Geometry: final body of the model. Coordinates: model frame, mm. Face numbers are marked on the shaded views. A direction names the side the tool comes from. Round coordinates to 2 decimals unless told otherwise and drop trailing zeros. Loops run counter-clockwise (first coordinate to the right, second up) from the corner with the lowest first, then second, coordinate; pieces in that order, holes last. Notation, with made-up numbers: M -8,85.25 L 22,85.25 A15 ccw 22,95.25 Z; hole C -32.75,77.5 d7. An arc over 180 degrees is marked long. Answer as a JSON object with one key per item and string values.
from build123d import *

# Parameters (mm, degrees)
BASPROSKE_W         = 4
BASPROSKE_H         = 22.5
TOOTHCUT_DEPTH      = 33.070235422
TEETHCUTS_COUNT     = 18
TEETHCUTS_ANGLE     = 340
BORSKE_R            = 1.5
BORE_DEPTH          = 50.0000508
SKETCH_1_R          = 1.5
CUT_EXTRUDE_1_DEPTH = 32.895398001


with BuildPart() as part:
    # BasProSke → Base-Revolve (revolve)
    with BuildSketch(Plane(origin=(0, 0, 0), x_dir=(1, 0, 0), z_dir=(0, 1, 0)), mode=Mode.PRIVATE) as base_revolve_sk:
        with Locations((2, 11.25)):
            Rectangle(BASPROSKE_W, BASPROSKE_H)
    revolve(base_revolve_sk.sketch.rotate(Axis((-10, 0, 0), (1, 0, 0)), 180), axis=Axis((-10, 0, 0), (1, 0, 0)))

    # TooCutSke → ToothCut (cut, through all)
    with BuildSketch(Plane(origin=(0, 0, 0), x_dir=(0, 0, -1), z_dir=(1, 0, 0))):
        with BuildLine():
            ThreePointArc((1.136237076, 17.399439576), (0, 17.4365), (-1.136237076, 17.399439576))
            ThreePointArc((-1.136237076, 17.399439576), (-1.836299497, 20.025700007), (-3.36570362, 22.272532059))
            ThreePointArc((-3.36570362, 22.272532059), (0, 22.5254), (3.36570362, 22.272532059))
            ThreePointArc((3.36570362, 22.272532059), (1.836299497, 20.025700007), (1.136237076, 17.399439576))
        make_face()
    toothcut = extrude(amount=TOOTHCUT_DEPTH, mode=Mode.SUBTRACT)

    # TeethCuts: ToothCut ×18 about axis
    teethcuts_axis = Axis((-10, 0, 0), (1, 0, 0))
    for i in range(1, TEETHCUTS_COUNT):
        add(toothcut.rotate(teethcuts_axis, i * TEETHCUTS_ANGLE / (TEETHCUTS_COUNT - 1)), mode=Mode.SUBTRACT)

    # BorSke → Bore (cut, symmetric)
    with BuildSketch(Plane(origin=(0, 0, 0), x_dir=(0, 0, -1), z_dir=(1, 0, 0))):
        with Locations(Location((0, 0, 0), (0, 0, 180))):
            Circle(BORSKE_R)
    extrude(amount=BORE_DEPTH, both=True, mode=Mode.SUBTRACT)

    # 草图1 → 切除-拉伸1 (cut, through all)
    with BuildSketch(Plane(origin=(4, 0, 0), x_dir=(0, 0, -1), z_dir=(1, 0, 0))):
        with Locations((0, 7)):
            Circle(SKETCH_1_R)
        with Locations((7, 0)):
            Circle(SKETCH_1_R)
        with Locations((-7, 0)):
            Circle(SKETCH_1_R)
        with Locations((0, -7)):
            Circle(SKETCH_1_R)
    extrude(amount=-CUT_EXTRUDE_1_DEPTH, mode=Mode.SUBTRACT)


solid = part.part
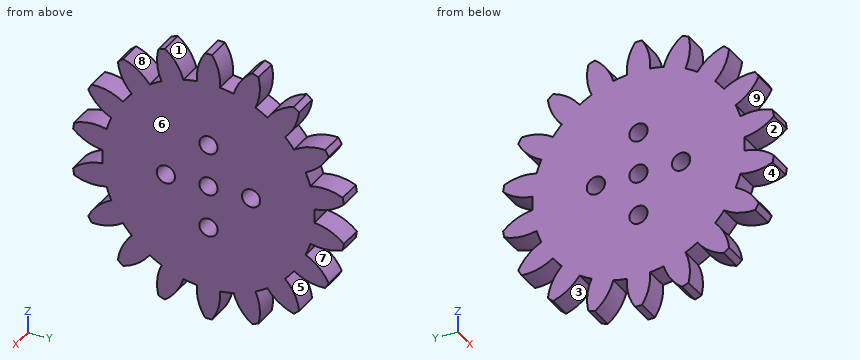
1) Reachability of the marked faces 1, 2, 3, 4 and 5 from +Z, -Z, +X, -X, +Y, -Y: full face, straight path, thin tool, end or side. Return the list, or none.
Results:
{"face 1": "+Z, +X, -X", "face 2": "+X, -X, -Y", "face 3": "-Z, +X, -X", "face 4": "+X, -X", "face 5": "+X, -X, +Y"}
2) Ray query, line 1 (Y direction, x = 2.95, z = 0); line 2 (Z direction, x = 3.8, y = -18.5); line 3 (Z direction, x = 2.1, y = -14). Return the intervals inside material, ascending.
Results:
{"line 1": "-17.44 to -8.5, -5.5 to -1.5, 1.5 to 5.5, 8.5 to 17.44", "line 2": "-11.76 to -8.9, -5.14 to -1.31, 1.31 to 5.14, 8.9 to 11.76", "line 3": "-17.59 to -13.96, -10.39 to 10.39, 13.96 to 17.59"}
3) Section query B-B (y = 0). Return the cut outline in (x, z), and give its area (3 significant figures).
Results:
{"outline": "M 0,-22.5 L 4,-22.5 L 4,-8.5 L 0,-8.5 Z; M 0,-5.5 L 4,-5.5 L 4,-1.5 L 0,-1.5 Z; M 0,1.5 L 4,1.5 L 4,5.5 L 0,5.5 Z; M 0,8.5 L 4,8.5 L 4,22.5 L 0,22.5 Z", "area": "144 mm2"}
4) Section query A-A (z = 0). Return the cut outline in (x, y), and give its area (3 significant figures).
Results:
{"outline": "M 0,-17.44 L 4,-17.44 L 4,-8.5 L 0,-8.5 Z; M 0,-5.5 L 4,-5.5 L 4,-1.5 L 0,-1.5 Z; M 0,1.5 L 4,1.5 L 4,5.5 L 0,5.5 Z; M 0,8.5 L 4,8.5 L 4,17.44 L 0,17.44 Z", "area": "103 mm2"}
5) Pull-direction query (Z, two-part tool) for the marked faces 6, 7, 8 and 9; classes: +Z half, -Z half, draft (parallel to the pull), parting line (faces both ways), or undercut.
Results:
{"face 6": "draft", "face 7": "undercut", "face 8": "+Z half", "face 9": "undercut"}
6) Pin query (flat end, axial travel): P1, Ø2, axis at x = 2, y = -12, coming from the -Z side; P2, Ø5, axis at y = 0, z = 0, coming from the +X side; P3, Ø2.5, axis at y = 0, z = -7, coming from the +X side; P4, Ø2, axis at x = 1.5, z = -8, coming from the +Y side. Return the tip coordinate at first contact, or that it passes through.
Results:
{"P1": "z = -17.22", "P2": "x = 4", "P3": "through", "P4": "y = 18.59"}
7) Section query C-C (x = 2.25). Count the separate pieces of the cut face and the enclosed holes in it, and give its area (3 significant figures).
Results:
{"separate pieces": "1", "enclosed holes": "5", "area": "1,200 mm2"}
